The listing builds one solid part. Answer for the finished solid, in the listing's coordinates (mm). A direction names the side the tool comes from. Give positions to 0.01 mm unless a question says otherwise; leave off trailing zeros. Write each loop counter-clockwise with the first axis right and the second up, starting at its lowest first coordinate (ties: lowest second). Pieces come first, ordered by that corner, then holes. Notation, with made-up numbers: (19.5, 28) - (27.5, 28) arc R21 ccw to (27.5, 35) - close; hole circle Ø5 at (-17, 36.5). An arc over 180 degrees is marked (long way). Answer in a Markdown table with one row per item. Add a question column.
Autodesk Inventor part; units mm, degrees
ref_plane "YZ Plane" through (0, 0, 0) normal (1, 0, 0) x (0, 1, 0)
ref_plane "XZ Plane" through (0, 0, 0) normal (0, 1, 0) x (-1, 0, 0)
ref_plane "XY Plane" through (0, 0, 0) normal (0, 0, 1) x (1, 0, 0)
sketch "Sketch1" plane through (0, 0, 0) normal (0, 1, 0) x (-1, 0, 0)
  line L0 (0, 0) -> (800, 0)
  line L1 (800, 0) -> (800, -800)
  line L2 (800, -800) -> (0, -800)
  line L3 (0, -800) -> (0, 0)
  line L4 (0, 0) -> (32.14, 0)
  line L5 (32.14, 0) -> (32.14, -800)
  line L6 (32.14, -800) -> (0, -800)
  line L7 (0, -800) -> (0, 0)
  line L8 (32.14, 0) -> (51.19, 0)
  line L9 (51.19, 0) -> (51.19, -800)
  line L10 (51.19, -800) -> (32.14, -800)
  line L11 (32.14, -800) -> (32.14, 0)
  line L12 (51.19, 0) -> (83.33, 0)
  line L13 (83.33, 0) -> (83.33, -800)
  line L14 (83.33, -800) -> (51.19, -800)
  line L15 (51.19, -800) -> (51.19, 0)
  line L16 (83.33, 0) -> (102.38, 0)
  line L17 (102.38, 0) -> (102.38, -800)
  line L18 (102.38, -800) -> (83.33, -800)
  line L19 (83.33, -800) -> (83.33, 0)
  line L20 (102.38, 0) -> (134.52, 0)
  line L21 (134.52, 0) -> (134.52, -800)
  line L22 (134.52, -800) -> (102.38, -800)
  line L23 (102.38, -800) -> (102.38, 0)
  line L24 (134.52, 0) -> (153.57, 0)
  line L25 (153.57, 0) -> (153.57, -800)
  line L26 (153.57, -800) -> (134.52, -800)
  line L27 (134.52, -800) -> (134.52, 0)
  line L28 (153.57, 0) -> (185.71, 0)
  line L29 (185.71, 0) -> (185.71, -800)
  line L30 (185.71, -800) -> (153.57, -800)
  line L31 (153.57, -800) -> (153.57, 0)
  line L32 (185.71, 0) -> (204.76, 0)
  line L33 (204.76, 0) -> (204.76, -800)
  line L34 (204.76, -800) -> (185.71, -800)
  line L35 (185.71, -800) -> (185.71, 0)
  line L36 (204.76, 0) -> (236.9, 0)
  line L37 (236.9, 0) -> (236.9, -800)
  line L38 (236.9, -800) -> (204.76, -800)
  line L39 (204.76, -800) -> (204.76, 0)
  line L40 (236.9, 0) -> (255.95, 0)
  line L41 (255.95, 0) -> (255.95, -800)
  line L42 (255.95, -800) -> (236.9, -800)
  line L43 (236.9, -800) -> (236.9, 0)
  line L44 (255.95, 0) -> (288.09, 0)
  line L45 (288.09, 0) -> (288.09, -800)
  line L46 (288.09, -800) -> (255.95, -800)
  line L47 (255.95, -800) -> (255.95, 0)
  line L48 (288.09, 0) -> (307.14, 0)
  line L49 (307.14, 0) -> (307.14, -800)
  line L50 (307.14, -800) -> (288.09, -800)
  line L51 (288.09, -800) -> (288.09, 0)
  line L52 (307.14, 0) -> (339.28, 0)
  line L53 (339.28, 0) -> (339.28, -800)
  line L54 (339.28, -800) -> (307.14, -800)
  line L55 (307.14, -800) -> (307.14, 0)
  line L56 (339.28, 0) -> (358.33, 0)
  line L57 (358.33, 0) -> (358.33, -800)
  line L58 (358.33, -800) -> (339.28, -800)
  line L59 (339.28, -800) -> (339.28, 0)
  line L60 (358.33, 0) -> (390.47, 0)
  line L61 (390.47, 0) -> (390.47, -800)
  line L62 (390.47, -800) -> (358.33, -800)
  line L63 (358.33, -800) -> (358.33, 0)
  line L64 (390.47, 0) -> (409.52, 0)
  line L65 (409.52, 0) -> (409.52, -800)
  line L66 (409.52, -800) -> (390.47, -800)
  line L67 (390.47, -800) -> (390.47, 0)
  line L68 (409.52, 0) -> (441.66, 0)
  line L69 (441.66, 0) -> (441.66, -800)
  line L70 (441.66, -800) -> (409.52, -800)
  line L71 (409.52, -800) -> (409.52, 0)
  line L72 (441.66, 0) -> (460.71, 0)
  line L73 (460.71, 0) -> (460.71, -800)
  line L74 (460.71, -800) -> (441.66, -800)
  line L75 (441.66, -800) -> (441.66, 0)
  line L76 (460.71, 0) -> (492.85, 0)
  line L77 (492.85, 0) -> (492.85, -800)
  line L78 (492.85, -800) -> (460.71, -800)
  line L79 (460.71, -800) -> (460.71, 0)
  line L80 (492.85, 0) -> (511.9, 0)
  line L81 (511.9, 0) -> (511.9, -800)
  line L82 (511.9, -800) -> (492.85, -800)
  line L83 (492.85, -800) -> (492.85, 0)
  line L84 (511.9, 0) -> (544.04, 0)
  line L85 (544.04, 0) -> (544.04, -800)
  line L86 (544.04, -800) -> (511.9, -800)
  line L87 (511.9, -800) -> (511.9, 0)
  line L88 (544.04, 0) -> (563.09, 0)
  line L89 (563.09, 0) -> (563.09, -800)
  line L90 (563.09, -800) -> (544.04, -800)
  line L91 (544.04, -800) -> (544.04, 0)
  line L92 (563.09, 0) -> (595.23, 0)
  line L93 (595.23, 0) -> (595.23, -800)
  line L94 (595.23, -800) -> (563.09, -800)
  line L95 (563.09, -800) -> (563.09, 0)
  line L96 (595.23, 0) -> (614.28, 0)
  line L97 (614.28, 0) -> (614.28, -800)
  line L98 (614.28, -800) -> (595.23, -800)
  line L99 (595.23, -800) -> (595.23, 0)
  line L100 (614.28, 0) -> (646.42, 0)
  line L101 (646.42, 0) -> (646.42, -800)
  line L102 (646.42, -800) -> (614.28, -800)
  line L103 (614.28, -800) -> (614.28, 0)
  line L104 (646.42, 0) -> (665.47, 0)
  line L105 (665.47, 0) -> (665.47, -800)
  line L106 (665.47, -800) -> (646.42, -800)
  line L107 (646.42, -800) -> (646.42, 0)
  line L108 (665.47, 0) -> (697.61, 0)
  line L109 (697.61, 0) -> (697.61, -800)
  line L110 (697.61, -800) -> (665.47, -800)
  line L111 (665.47, -800) -> (665.47, 0)
  line L112 (697.61, 0) -> (716.66, 0)
  line L113 (716.66, 0) -> (716.66, -800)
  line L114 (716.66, -800) -> (697.61, -800)
  line L115 (697.61, -800) -> (697.61, 0)
  line L116 (716.66, 0) -> (748.8, 0)
  line L117 (748.8, 0) -> (748.8, -800)
  line L118 (748.8, -800) -> (716.66, -800)
  line L119 (716.66, -800) -> (716.66, 0)
  line L120 (748.8, 0) -> (767.85, 0)
  line L121 (767.85, 0) -> (767.85, -800)
  line L122 (767.85, -800) -> (748.8, -800)
  line L123 (748.8, -800) -> (748.8, 0)
  dimension "d0" = 800
  dimension "d1" = 800
  dimension "d2" = 32.14
  dimension "d4" = 19.05
  dimension "d6" = 32.14
  dimension "d7" = 19.05
  dimension "d8" = 32.14
  dimension "d9" = 19.05
  dimension "d10" = 32.14
  dimension "d11" = 19.05
  dimension "d12" = 32.14
  dimension "d13" = 19.05
  dimension "d14" = 32.14
  dimension "d15" = 19.05
  dimension "d16" = 32.14
  dimension "d17" = 19.05
  dimension "d18" = 32.14
  dimension "d19" = 19.05
  dimension "d20" = 32.14
  dimension "d21" = 19.05
  dimension "d22" = 32.14
  dimension "d23" = 19.05
  dimension "d24" = 32.14
  dimension "d25" = 19.05
  dimension "d26" = 32.14
  dimension "d27" = 19.05
  dimension "d28" = 32.14
  dimension "d29" = 19.05
  dimension "d30" = 32.14
  dimension "d31" = 19.05
  dimension "d32" = 32.14
  dimension "d33" = 19.05
extrude "Extrusion1" add sketch "Sketch1" along normal blind 1 contours L0 L5 L2 L3 | L0 L13 L2 L9 | L0 L21 L2 L17 | L0 L29 L2 L25 | L0 L37 L2 L33 | L0 L45 L2 L41 | L0 L53 L2 L49 | L0 L61 L2 L57 | L0 L69 L2 L65 | L0 L77 L2 L73 | L0 L85 L2 L81 | L0 L93 L2 L89 | L0 L101 L2 L97 | L0 L109 L2 L105 | L0 L117 L2 L113 | L0 L1 L2 L121
extrude "Extrusion2" add sketch "Sketch1" along normal blind 2 contours L0 L9 L2 L5 | L0 L17 L2 L13 | L0 L25 L2 L21 | L0 L33 L2 L29 | L0 L41 L2 L37 | L0 L49 L2 L45 | L0 L57 L2 L53 | L0 L65 L2 L61 | L0 L73 L2 L69 | L0 L81 L2 L77 | L0 L89 L2 L85 | L0 L97 L2 L93 | L0 L105 L2 L101 | L0 L113 L2 L109 | L0 L121 L2 L117
properties part number "Sensor Grid Rows-Collumns"
1. The mould has two halves that part along X. Classify faces 1 (the face through (-169, 1, -394)), 2 (the face through (-502, 2, -394)): +X half, -X half, draft (parallel to the pull), parting line (faces both ways), or undercut.
2. A tool of negligible diameter and unlimited length cuts with its end or side. For faces 3 (the face through (-477, 1, -394)), 4 (the face through (-394, 0, -394)), 5 (the face through (-784, 1, -394)), from which of +Z, -Z, +X, -X, +Y, -Y can it reach the whole face along a straight path? Write none if from no direction.
3. Section A-A (y = 1.65) is taken. State how many separate pieces and enclosed holes the cut face has, and give its area (3 significant figures).
4. A straight line is drawn through the part: L1, parallel to Y at x = -413, z = -418. Find the intervals that lie inside material, in ascending order. Write a range as [from, to].
5. Given pin 1 Ø9.5 at (x, z) = (-425.5, -519.5) entering from +Y; pin 2 Ø0.8 at (y, z) = (1.5, -586) entering from +X; pin 3 Ø0.5 at (y, z) = (1.5, -494) entering from -X, each flat-ended and moving along its own axis, determine where each tip first touches the part or whether it passes through.
6. Section B-B (x = -317) is taken. Give the vertices of the cut face in (y, z).
Geometry check:
| question | item | result |
|---|---|---|
| 1 | face 1 | undercut |
| 1 | face 2 | draft |
| 2 | face 3 | +Z, -Z, +Y |
| 2 | face 4 | +Z, -Z, +X, -X, -Y |
| 2 | face 5 | +Z, -Z, -X, +Y |
| 3 | separate pieces | 15 |
| 3 | enclosed holes | 0 |
| 3 | area | 229,000 mm² |
| 4 | L1 | [0, 1] |
| 5 | pin 1 | y = 1 |
| 5 | pin 2 | x = -32.14 |
| 5 | pin 3 | x = -767.85 |
| 6 | outline | (0, -800) - (1, -800) - (1, 0) - (0, 0) - close |
